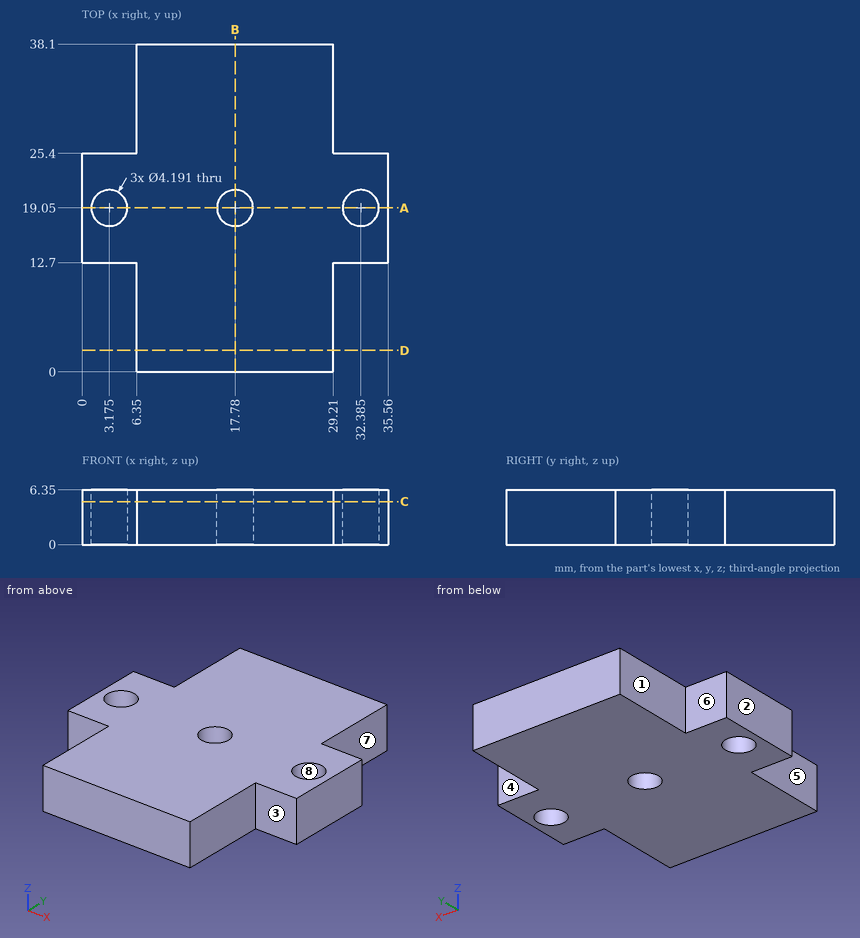
Can you work these out from the drawing? Everything is in mm from the part's minimum corner. A direction names the side the tool comes from. Round coordinates to 2 decimals unless told otherwise and drop trailing zeros. Loops run counter-clockwise (first coordinate to the right, second up) from the corner with the lowest first, then second, coordinate; pieces in that order, holes last. Notation, with made-up numbers: (10.5, -21) -> (43.5, -21) arc R28 ccw to (43.5, 5) -> close; hole circle Ø8 at (61.5, 80.25). An arc over 180 degrees is marked (long way). One line per question, with ' | ' between items.
(1) Thinking about a two-plate mould opening in X: for the marked faces 6, 7 and 8, which applies, released by +X, released by -X, zero draft, split by the parting line, or undercut?
Model answer:
face 6: zero draft | face 7: released by +X | face 8: undercut
(2) If we section it at D-D on y = 2.5: List the corners of the cut face in (x, z) for me, and give its area (3 significant figures).
Model answer:
outline: (6.35, 0) -> (29.21, 0) -> (29.21, 6.35) -> (6.35, 6.35) -> close | area: 145 mm^2
(3) If I drill on probe 1 along X at (y, z) = (19, 5.75); probe 2 along Y at (x, z) = (17.78, 2); probe 3 along Y at (x, z) = (32.5, 4.75), over which ranges is the centre line in solid material (lowest first)?
Model answer:
probe 1: x = 0 to 1.08, 5.27 to 15.69, 19.87 to 30.29, 34.48 to 35.56 | probe 2: y = 0 to 16.95, 21.15 to 38.1 | probe 3: y = 12.7 to 16.96, 21.14 to 25.4
(4) If we section it at C-C on z = 5: Count the separate pieces of the cut face and the enclosed holes in it, and give its area (3 significant figures).
Model answer:
separate pieces: 1 | enclosed holes: 3 | area: 991 mm^2
(5) For the marked faces 1, 2, 3, 4 and 5, which set-ups out of +Z, -Z, +X, -X, +Y, -Y let a thin tool reach every point of the face, with its end or its side?
Model answer:
face 1: +Z, -Z, -X, +Y | face 2: +Z, -Z, -X, +Y, -Y | face 3: +Z, -Z, +X, -Y | face 4: +Z, -Z, +X, +Y | face 5: +Z, -Z, -X, -Y
(6) If we section it at A-A on y = 19.05: List the corners of the cut face in (x, z) for me.
Model answer:
outline: (0, 0) -> (1.08, 0) -> (1.08, 6.35) -> (0, 6.35) -> close; (5.27, 0) -> (15.68, 0) -> (15.68, 6.35) -> (5.27, 6.35) -> close; (19.88, 0) -> (30.29, 0) -> (30.29, 6.35) -> (19.88, 6.35) -> close; (34.48, 0) -> (35.56, 0) -> (35.56, 6.35) -> (34.48, 6.35) -> close
(7) If we section it at B-B on x = 17.78: List the corners of the cut face in (y, z) for me, and give its area (3 significant figures).
Model answer:
outline: (0, 0) -> (16.95, 0) -> (16.95, 6.35) -> (0, 6.35) -> close; (21.15, 0) -> (38.1, 0) -> (38.1, 6.35) -> (21.15, 6.35) -> close | area: 215 mm^2
(8) For pin 1 Ø1.9 at (y, z) = (28.5, 3) entering from -X; pin 2 Ø1 at (y, z) = (10, 4) entering from +X; pin 3 Ø1.9 at (x, z) = (2.5, 2) entering from +Y, each with a flat end and sliding along its axis, tell me the tip position at first contact or that it passes through.
Model answer:
pin 1: stops at x = 6.35 | pin 2: stops at x = 29.21 | pin 3: stops at y = 25.4
